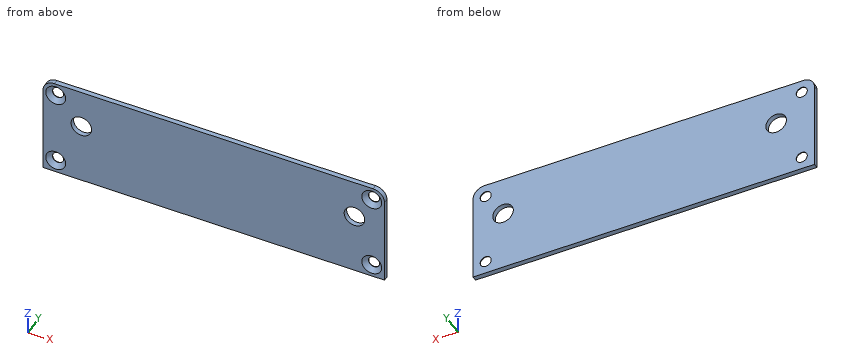
from build123d import *

# Parameters (mm, degrees)
SKETCH_W            = 104.8
SKETCH_H            = 31
PAD_DEPTH           = 1.5
HOLE_D              = 3.4
HOLE_DEPTH          = 25
HOLE_CSINK_D        = 6.1
HOLE_CSINK_ANGLE    = 90
FILLET_R            = 3.5
SKETCH002_R         = 3.15
POCKET_DEPTH        = 1.501
LINEARPATTERN_COUNT = 2
LINEARPATTERN_PITCH = 83.82


with BuildPart() as part:
    # Sketch → Pad (new body)
    with BuildSketch(Plane.XZ):
        Rectangle(SKETCH_W, SKETCH_H)
    extrude(amount=PAD_DEPTH)

    # Hole
    with Locations(Plane.XZ.offset(1.5)):
        with Locations((-48.5, 11.5), (-48.5, -11.5), (48.5, -11.5), (48.5, 11.5)):
            CounterSinkHole(HOLE_D / 2, HOLE_CSINK_D / 2, depth=HOLE_DEPTH, counter_sink_angle=HOLE_CSINK_ANGLE)

    # Fillet
    fillet_edges = [part.edges().sort_by_distance(p)[0] for p in [
        (-52.4, -0.75, 15.5),
        (52.4, -0.75, 15.5),
    ]]
    fillet(fillet_edges, radius=FILLET_R)

    # Sketch002 (on Face5 of Fillet) → Pocket (cut, through all)
    with BuildSketch(Plane.XZ.offset(1.5)):
        with Locations((-40.64, 3.52)):
            Circle(SKETCH002_R)
    pocket = extrude(amount=-POCKET_DEPTH, mode=Mode.SUBTRACT)

    # LinearPattern: Pocket ×2
    with Locations(*[(i * LINEARPATTERN_PITCH, 0, 0) for i in range(1, LINEARPATTERN_COUNT)]):
        add(pocket, mode=Mode.SUBTRACT)


solid = part.part
Source: CAD feature listing. Evaluate the final solid. Frame: model axes, mm. Coordinates: 2 decimals unless noted, no trailing zeros. Order: outer loops, then holes, each group sorted by start corner. A loop starts at its lowest first (then second) coordinate and runs counter-clockwise, first axis right, second up. Notation, with made-up numbers: M -13,5 L 32,5 A24 ccw 32,22 Z; hole C -40,-26 d1. An arc over 180 degrees is marked long. Write each question's results on one line, items separated by ' | '. Start each with the question number.
Item 1: Cut plane C-C (x = -40.64). Return loops of the section in (y, z), and give its area (4 significant figures).
Item 2: Cut plane B-B (y = -0.8). Return loops of the section in (x, z).
Item 3: First-contact query: pin 1 Ø5.5 at (x, z) = (48.5, -11.5) entering from -Y. Flat tip, straight axial feed; report the tip coordinate or a pass-through.
Item 4: Line query: probe 1 along Z at (x, y) = (48.5, -0.1); probe 2 along X at (y, z) = (-0.9, 3.5); probe 3 along X at (y, z) = (-0.05, 11.5). Output: solid intervals per line, ascending.
Item 5: Cut plane A-A (z = -11.5). Return loops of the section in (x, y).
Checked values:
1) outline: M -1.5,-15.5 L 0,-15.5 L 0,0.37 L -1.5,0.37 Z; M -1.5,6.67 L 0,6.67 L 0,15.5 L -1.5,15.5 Z | area: 37.05 mm2
2) outline: M -52.4,-15.5 L 52.4,-15.5 L 52.4,12 A3.5 ccw 48.9,15.5 L -48.9,15.5 A3.5 ccw -52.4,12 Z; hole C -48.5,-11.5 d4.7; hole C -48.5,11.5 d4.7; hole C -40.64,3.52 d6.3; hole C 43.18,3.52 d6.3; hole C 48.5,-11.5 d4.7; hole C 48.5,11.5 d4.7
3) pin 1: stops at y = -1.2
4) probe 1: z = -15.5 to -13.2, -9.8 to 9.8, 13.2 to 15.5 | probe 2: x = -52.4 to -43.79, -37.49 to 40.03, 46.33 to 52.4 | probe 3: x = -52.4 to -50.2, -46.8 to 46.8, 50.2 to 52.4
5) outline: M -52.4,-1.5 L -51.55,-1.5 L -50.2,-0.15 L -50.2,0 L -52.4,0 Z; M -46.8,-0.15 L -45.45,-1.5 L 45.45,-1.5 L 46.8,-0.15 L 46.8,0 L -46.8,0 Z; M 50.2,-0.15 L 51.55,-1.5 L 52.4,-1.5 L 52.4,0 L 50.2,0 Z
